Autodesk Inventor part; units mm, degrees
ref_plane "YZ Plane" through (0, 0, 0) normal (1, 0, 0) x (0, 1, 0)
ref_plane "XZ Plane" through (0, 0, 0) normal (0, 1, 0) x (-1, 0, 0)
ref_plane "XY Plane" through (0, 0, 0) normal (0, 0, 1) x (1, 0, 0)
sketch "스케치1" plane through (0, 0, 0) normal (0, 1, 0) x (-1, 0, 0)
  line L0 (0, 0) -> (16, 0)
  line L1 (16, 0) -> (16, -17.5)
  line L2 (16, -17.5) -> (0, -17.5)
  line L3 (0, -17.5) -> (0, 0)
  dimension "d0" = 16
  dimension "d1" = 17.5
extrude "돌출1" add sketch "스케치1" along normal blind 1
sketch "스케치2" plane through (0, 1, 0) normal (0, 1, 0) x (1, 0, 0)
  line L0 (-16, 0) -> (0, 0)
  line L1 (0, 0) -> (0, 17.5)
  line L2 (0, 17.5) -> (-16, 17.5)
  line L3 (-16, 17.5) -> (-16, 0)
  line L4 (-16, 0) -> (0, 0)
  line L5 (-16, 17.5) -> (-14.5, 17.5)
  line L6 (-14.5, 17.5) -> (-14.5, 0)
  line L7 (-14.5, 0) -> (-16, 0)
  line L8 (-16, 0) -> (-16, 17.5)
  line L9 (0, 17.5) -> (-16, 17.5)
  line L10 (0, 0) -> (-1.5, 0)
  line L11 (-1.5, 0) -> (-1.5, 17.5)
  line L12 (-1.5, 17.5) -> (0, 17.5)
  line L13 (0, 17.5) -> (0, 0)
  point P0 (-1.5, 0)
  point P1 (-14.5, 0)
  dimension "d4" = 1.5
  dimension "d5" = 1.5
extrude "돌출2" add sketch "스케치2" along normal blind 3 contours L3 L2 L6 L0 | L11 L2 L1 L0
chamfer "모따기1" distance 1 distance2 3 1 edges at (0, 4, -8.75) measured on face at (-1, 4, -11.6667)
chamfer "모따기2" distance 1 distance2 3 1 edges at (-16, 4, -8.75) measured on face at (-15, 4, -5.8333)
fillet "모깎기1" radius 2 2 edges at (-16, 0, -8.75) (0, 0, -8.75)
properties part number "_3D 인쇄"
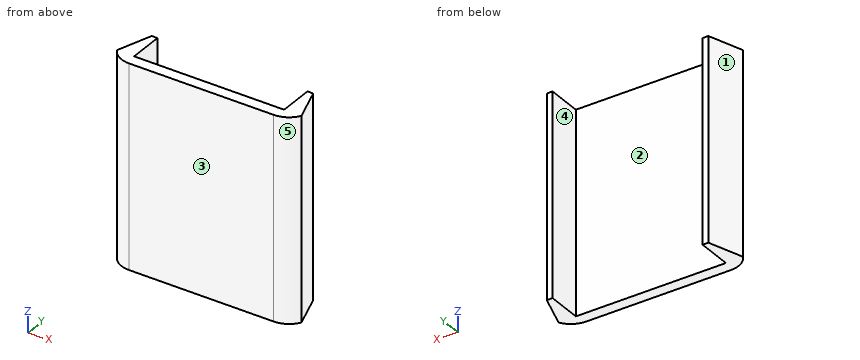
Geometry: final body of the model. Coordinates: model frame, mm. Face numbers are marked on the shaded views. A direction names the side the tool comes from. Coordinates: 2 decimals unless noted, no trailing zeros. Loops run counter-clockwise (first coordinate to the right, second up) from the corner with the lowest first, then second, coordinate; pieces in that order, holes last. Notation, with made-up numbers: (0.25, 72.25) -> (53.25, 72.25) arc R23 ccw to (53.25, 97.25) -> close; hole circle Ø4 at (-39, 72.25). An arc over 180 degrees is marked (long way). Use a Markdown table: item, result. Add a question column.
(1) Section query D-D, the plane x = -5.5. Return loops of the section in (y, z).
(2) Section query A-A, the plane y = 3.6. Return loops of the section in (x, z), plus the area to 3 significant figures.
(3) Line query: line 1 along Y through (x, z) = (-5.25, -15); line 2 along X through (y, z) = (2.25, -16.5); line 3 along X through (y, z) = (3.8, -12.25). Output: solid intervals per line, ascending.
(4) Pin query (flat end, axial travel): pin 1 Ø1.5 at (y, z) = (3, -9.5) entering from +X. Return the tip coordinate at first contact, or that it passes through.
(5) Section query C-C, the plane y = 1.5. Return loops of the section in (x, z), plus the area to 3 significant figures.
(6) Section query B-B, the plane z = -11.5. Return loops of the section in (x, y), plus the area to 3 significant figures.
(7) Access query for the marked faces 1 and 2. Directions: +Z, -Z, +X, -X, +Y, -Y. A direction counts if a zero-diameter tool reaches every point of the face in a straight line with its end or side. Return the directions, or none.
(8) Mould query, pull axis X, two halves, no side actions, for the marked faces 3, 4 and 5. Classes: pulls with the +X half, pulls with the -X half, needs draft (parallel to the pull), parting line crosses it, or undercut.
Answer:
| question | item | result |
|---|---|---|
| 1 | outline | (0, -17.5) -> (1, -17.5) -> (1, 0) -> (0, 0) -> close |
| 2 | outline | (-15.13, -17.5) -> (-14.5, -17.5) -> (-14.5, 0) -> (-15.13, 0) -> close; (-1.5, -17.5) -> (-0.87, -17.5) -> (-0.87, 0) -> (-1.5, 0) -> close |
| 2 | area | 22.2 mm^2 |
| 3 | line 1 | y = 0 to 1 |
| 3 | line 2 | x = -15.58 to -14.5, -1.5 to -0.42 |
| 3 | line 3 | x = -15.07 to -14.5, -1.5 to -0.93 |
| 4 | pin 1 | stops at x = -0.42 |
| 5 | outline | (-15.83, -17.5) -> (-14.5, -17.5) -> (-14.5, 0) -> (-15.83, 0) -> close; (-1.5, -17.5) -> (-0.17, -17.5) -> (-0.17, 0) -> (-1.5, 0) -> close |
| 5 | area | 46.7 mm^2 |
| 6 | outline | (-16, 1) arc R2 ccw to (-14.27, 0) -> (-1.73, 0) arc R2 ccw to (0, 1) -> (-1, 4) -> (-1.5, 4) -> (-1.5, 1) -> (-14.5, 1) -> (-14.5, 4) -> (-15, 4) -> close |
| 6 | area | 21.0 mm^2 |
| 7 | face 1 | +Z, -Z, -X, +Y |
| 7 | face 2 | +Z, -Z, +Y |
| 8 | face 3 | needs draft |
| 8 | face 4 | undercut |
| 8 | face 5 | pulls with the +X half |
